Geometry: final body of the model. Coordinates: model frame, mm. A direction names the side the tool comes from. Round coordinates to 2 decimals unless told otherwise and drop trailing zeros. Loops run counter-clockwise (first coordinate to the right, second up) from the corner with the lowest first, then second, coordinate; pieces in that order, holes last. Notation, with made-up numbers: M -37.75,-32 L 15.25,-32 A7 cw 15.25,-24 Z; hole C -1,17.25 d3. An arc over 180 degrees is marked long. Answer as a JSON object with one key per item and string values.
```python
from build123d import *

# Parameters (mm, degrees)
SKETCH1_R                       = 6.35
BOSS_EXTRUDE1_DEPTH             = 76.2
SKETCH8_R                       = 1.3208
CUT_EXTRUDE1_DEPTH              = 77.2
SKETCH10_R                      = 6.35
SKETCH10_R_2                    = 4.7625
CUT_EXTRUDE2_DEPTH              = 12.7
F_1_4_0_25_DIAMETER_HOLE1_D     = 6.35
F_1_4_0_25_DIAMETER_HOLE1_DEPTH = 63.5
F_1_4_0_25_DIAMETER_HOLE1_TIP   = 1.907732465


with BuildPart() as part:
    # Sketch1 → Boss-Extrude1 (new body)
    with BuildSketch(Plane.XY):
        Circle(SKETCH1_R)
    extrude(amount=BOSS_EXTRUDE1_DEPTH)

    # Sketch7 → Cut-Revolve1 (revolve, cut)
    with BuildSketch(Plane(origin=(0, 0, 0), x_dir=(1, 0, 0), z_dir=(0, 1, 0))):
        Polygon((6.35, -76.2), (6.35, -50.991152312), (1.905, -76.2), align=None)
    revolve(axis=Axis((0, 0, -47.573976859), (0, 0, 1)), mode=Mode.SUBTRACT)

    # Sketch8 → Cut-Extrude1 (cut, through all)
    with BuildSketch(Plane.XY.offset(76.2)):
        Circle(SKETCH8_R)
    extrude(amount=-CUT_EXTRUDE1_DEPTH, mode=Mode.SUBTRACT)

    # Sketch10 → Cut-Extrude2 (cut)
    with BuildSketch(Plane(origin=(0, 0, 0), x_dir=(-1, 0, 0), z_dir=(0, 0, -1))):
        Circle(SKETCH10_R)
        Circle(SKETCH10_R_2, mode=Mode.SUBTRACT)
    extrude(amount=-CUT_EXTRUDE2_DEPTH, mode=Mode.SUBTRACT)

    # 1/4 (0.25) Diameter Hole1
    with Locations(Plane(origin=(0, 0, 0), x_dir=(-1, 0, 0), z_dir=(0, 0, -1))):
        with Locations((0, 0)):
            Hole(F_1_4_0_25_DIAMETER_HOLE1_D / 2, depth=F_1_4_0_25_DIAMETER_HOLE1_DEPTH)
            with Locations((0, 0, -(F_1_4_0_25_DIAMETER_HOLE1_DEPTH + F_1_4_0_25_DIAMETER_HOLE1_TIP / 2))):  # 118° drill point
                Cone(0, F_1_4_0_25_DIAMETER_HOLE1_D / 2, F_1_4_0_25_DIAMETER_HOLE1_TIP, mode=Mode.SUBTRACT)

    # Sketch18 → Cut-Revolve2 (revolve, cut)
    with BuildSketch(Plane(origin=(0, 0, 0), x_dir=(1, 0, 0), z_dir=(0, 1, 0))):
        with BuildLine():
            Line((4.7625, -12.7), (4.1656, -12.7))
            ThreePointArc((4.1656, -12.7), (3.6576, -12.192), (4.1656, -11.684))
            Line((4.1656, -11.684), (4.7625, -11.684))
            Line((4.7625, -11.684), (4.7625, -12.7))
        make_face()
    revolve(axis=Axis((0, 0, 0.466216552), (0, 0, -1)), mode=Mode.SUBTRACT)

    # Sketch20 → Cut-Revolve3 (revolve, cut)
    with BuildSketch(Plane(origin=(0, 0, 0), x_dir=(1, 0, 0), z_dir=(0, 1, 0))):
        Polygon((4.7625, 0), (4.7625, -1.2319), (3.5306, 0), align=None)
    revolve(axis=Axis((0, 0, 0.466216552), (0, 0, -1)), mode=Mode.SUBTRACT)


solid = part.part
```
1) First-contact query: pin 1 (3 mm diameter, centred on x = 0, y = 0, fed in from -Z); pin 2 (6 mm diameter, centred on x = -2, z = 25.5, fed in from +Y); pin 3 (1 mm diameter, centred on y = 2, z = 46, fed in from -X); pin 4 (4 mm diameter, centred on x = -3.5, z = 53, fed in from -Y). Flat tips, straight axial feed; report the tip coordinate or a pass-through.
Geometry results:
{"pin 1": "z = 64.51", "pin 2": "y = 6.35", "pin 3": "x = -6.17", "pin 4": "y = -5.91"}
2) Pull-direction query (Z, two-part tool) for faces 1 (the face through (-0.89, -4, 63.77)), 2 (the face through (-1.38, -6.2, 31.58)), 3 (the face through (-4.14, -1.32, 12.7)); classes: +Z half, -Z half, draft (parallel to the pull), parting line (faces both ways), or undercut.
Geometry results:
{"face 1": "+Z half", "face 2": "draft", "face 3": "undercut"}
3) Cut plane C-C on z = 29.5. Return the cut outline in (x, y) (3 decimals).
Geometry results:
{"outline": "C 0,0 d12.7; hole C 0,0 d6.35"}
4) Set-up query: faces 4 (the face through (-1.05, -0.8, 70.49)), 5 (the face through (-2, 4, 11.684)), 6 (the face through (-0.69, -3.1, 32.19)). Return all of +Z, -Z, +X, -X, +Y, -Y with unobstructed straight access to the full face (end or side cutting, diameter ignored); none if empty.
Geometry results:
{"face 4": "+Z, -Z", "face 5": "none", "face 6": "-Z"}
5) Line query: probe 1 along Y at (x, z) = (0, 69); probe 2 along Y at (x, z) = (0, 49.5) (3 decimals); probe 3 along Y at (x, z) = (-4.5, 54.5). Output: solid intervals per line, ascending.
Geometry results:
{"probe 1": "-3.17 to -1.32, 1.32 to 3.17", "probe 2": "-6.35 to -3.175, 3.175 to 6.35", "probe 3": "-3.55 to 3.55"}
